```python
from build123d import *

# Parameters (mm, degrees)
ESQUISSE1_R             = 16
ESQUISSE1_R_2           = 3.1
BOSS_EXTRU_1_DEPTH      = 6.7
ESQUISSE2_R             = 13.660407535
ESQUISSE2_R_2           = 7.85
ENL_V_MAT_EXTRU_1_DEPTH = 5.15
ESQUISSE4_R             = 10
ESQUISSE4_R_2           = 3.025
BOSS_EXTRU_2_DEPTH      = 7
ESQUISSE5_R             = 2
ENL_V_MAT_EXTRU_3_DEPTH = 17


with BuildPart() as part:
    # Esquisse1 → Boss.-Extru.1 (new body, symmetric)
    with BuildSketch(Plane.XY):
        Circle(ESQUISSE1_R)
        Circle(ESQUISSE1_R_2, mode=Mode.SUBTRACT)
    extrude(amount=BOSS_EXTRU_1_DEPTH, both=True)

    # Esquisse2 → Enlèv. mat.-Extru.1 (cut, symmetric)
    with BuildSketch(Plane.XY):
        Circle(ESQUISSE2_R)
        Circle(ESQUISSE2_R_2, mode=Mode.SUBTRACT)
    extrude(amount=ENL_V_MAT_EXTRU_1_DEPTH, both=True, mode=Mode.SUBTRACT)

    # Esquisse4 → Boss.-Extru.2 (add)
    with BuildSketch(Plane.XY.offset(6.7)):
        Circle(ESQUISSE4_R)
        Circle(ESQUISSE4_R_2, mode=Mode.SUBTRACT)
    extrude(amount=BOSS_EXTRU_2_DEPTH)

    # Esquisse5 → Enlèv. mat.-Extru.3 (cut, through all)
    with BuildSketch(Plane(origin=(0, 0, 0), x_dir=(1, 0, 0), z_dir=(0, 1, 0))):
        with Locations((0, -10.2)):
            Circle(ESQUISSE5_R)
    extrude(amount=ENL_V_MAT_EXTRU_3_DEPTH, mode=Mode.SUBTRACT)


solid = part.part
```
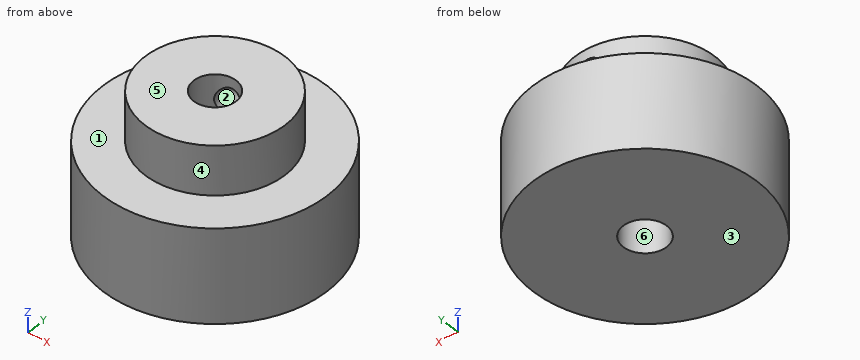
Design review of the part built by this model. Coordinates are the model's own, in mm. Face numbers are marked on the shaded views. A direction names the side the tool comes from. Round coordinates to 2 decimals unless told otherwise and drop trailing zeros. Write each loop counter-clockwise with the first axis right and the second up, starting at its lowest first coordinate (ties: lowest second). Pieces come first, ordered by that corner, then holes.
Item 1: For the marked faces 1, 2 and 3, list the 3-axis set-ups (+Z, -Z, +X, -X, +Y, -Y) from which the entire face can be reached by the end or side of a thin tool; tool diameter is ignored.
Item 2: Clearance check with flat-ended pins moving along their axes: pin 1 Ø1.9 at (x, y) = (-1.5, -1) entering from -Z; pin 2 Ø5 at (x, z) = (-8, 11) entering from +Y; pin 3 Ø10 at (x, z) = (7, 0.5) entering from +Y; pin 4 Ø2 at (x, z) = (-6, 8.5) entering from +Y. State where each tip first meets the part, or that it passes through.
Item 3: For probe 1 along Y at (x, z) = (0, -3); probe 2 along Z at (x, y) = (11, 7); probe 3 along Z at (x, y) = (0, 4), list the stretches that pass through material, from the lowest coordinate up.
Item 4: We need section A-A on y = 0. Write out the cut boundary in (x, z) (3 decimals).
Item 5: The part is to be moulded in two halves that separate along X. For the marked faces 4, 5 and 6, say which applies: +X half, -X half, draft (parallel to the pull), parting line (faces both ways), or undercut.
Item 6: We need section D-D on x = 9. Write out the cut boundary in (y, z), and give its area (3 significant figures).
Item 7: We need section C-C on x = -6. Write out the cut boundary in (y, z).
Item 8: We need section B-B on z = 1. Write out the cut boundary in (x, y), and give its area (3 significant figures).
Returned:
1. face 1: +Z
1. face 2: +Y
1. face 3: -Z, +X, -X, +Y, -Y
2. pin 1: passes through
2. pin 2: stops at y = 8.35
2. pin 3: stops at y = 15.87
2. pin 4: stops at y = 8.66
3. probe 1: y = -16 to -13.66, -7.85 to -3.1, 3.1 to 7.85, 13.66 to 16
3. probe 2: z = -6.7 to -5.15, 5.15 to 6.7
3. probe 3: z = -6.7 to 8.2, 12.2 to 13.7
4. outline: (-16, -6.7) - (-3.1, -6.7) - (-3.1, 6.7) - (-3.025, 6.7) - (-3.025, 13.7) - (-10, 13.7) - (-10, 6.7) - (-16, 6.7) - close; (3.025, 6.7) - (3.1, 6.7) - (3.1, -6.7) - (16, -6.7) - (16, 6.7) - (10, 6.7) - (10, 13.7) - (3.025, 13.7) - close; hole (-13.66, -5.15) - (-7.85, -5.15) - (-7.85, 5.15) - (-13.66, 5.15) - close; hole (7.85, -5.15) - (13.66, -5.15) - (13.66, 5.15) - (7.85, 5.15) - close
5. face 4: parting line
5. face 5: draft
5. face 6: undercut
6. outline: (-13.23, -6.7) - (13.23, -6.7) - (13.23, 6.7) - (4.36, 6.7) - (4.36, 13.7) - (-4.36, 13.7) - (-4.36, 6.7) - (-13.23, 6.7) - close; hole (-10.28, -5.15) - (10.28, -5.15) - (10.28, 5.15) - (-10.28, 5.15) - close
6. area: 204 mm2
7. outline: (-14.83, -6.7) - (14.83, -6.7) - (14.83, 6.7) - (8, 6.7) - (8, 13.7) - (-8, 13.7) - (-8, 6.7) - (-14.83, 6.7) - close; hole (-12.27, -5.15) - (-5.06, -5.15) - (-5.06, 5.15) - (-12.27, 5.15) - close; hole (5.06, -5.15) - (12.27, -5.15) - (12.27, 5.15) - (5.06, 5.15) - close
8. outline: circle Ø32 at (0, 0); circle Ø15.7 at (0, 0); hole circle Ø27.32 at (0, 0); hole circle Ø6.2 at (0, 0)
8. area: 381 mm2
